from build123d import *

# Parameters (mm, degrees)
SKETCH1_W             = 152.4
SKETCH1_H             = 38.1
BOSS_EXTRUDE1_DEPTH   = 6.35
CAVITY1_START         = -18.462835622
CAVITY1_OUTLINE_W     = 6.35
CAVITY1_OUTLINE_H     = 6.35
CAVITY1_OUTLINE_W_2   = 6.2484
CAVITY1_DEPTH         = 12.7
CAVITY1_START_2       = 6.937164378
CAVITY1_2_OUTLINE_W   = 6.35
CAVITY1_2_OUTLINE_H   = 6.35
CAVITY1_2_OUTLINE_W_2 = 6.2484
CAVITY1_2_DEPTH       = 12.7
CAVITY1_START_3       = 32.337164378
CAVITY1_3_OUTLINE_W   = 6.35
CAVITY1_3_OUTLINE_H   = 6.35
CAVITY1_3_OUTLINE_W_2 = 6.2484
CAVITY1_3_DEPTH       = 12.7
CAVITY1_START_4       = 57.737164378
CAVITY1_4_OUTLINE_W   = 6.35
CAVITY1_4_OUTLINE_H   = 6.35
CAVITY1_4_OUTLINE_W_2 = 6.2484
CAVITY1_4_DEPTH       = 12.7
CAVITY1_START_5       = 83.137164378
CAVITY1_5_OUTLINE_W   = 6.35
CAVITY1_5_OUTLINE_H   = 6.35
CAVITY1_5_OUTLINE_W_2 = 6.2484
CAVITY1_5_DEPTH       = 12.7
CAVITY1_START_6       = -37.512835622
CAVITY1_6_OUTLINE_W   = 9.525
CAVITY1_6_OUTLINE_H   = 6.35
CAVITY1_6_DEPTH       = 6.35
CAVITY1_START_7       = 108.537164378
CAVITY1_7_OUTLINE_W   = 9.525
CAVITY1_7_OUTLINE_H   = 6.35
CAVITY1_7_DEPTH       = 6.35
SKETCH2_R             = 7.9375
CUT_EXTRUDE1_DEPTH    = 166.74710148
LPATTERN1_COUNT       = 5
LPATTERN1_PITCH       = 25.4


# Read off the part's stored shape, not the designer's step: Cavity1
with BuildPart() as part:
    # Sketch1 → Boss-Extrude1 (new body)
    with BuildSketch(Plane.XY):
        with Locations((38.687164378, -100.250958128)):
            Rectangle(SKETCH1_W, SKETCH1_H)
    extrude(amount=BOSS_EXTRUDE1_DEPTH)

    # Cavity1 outline → Cavity1 (cut)
    with BuildSketch(Plane.YZ.offset(CAVITY1_START)):
        with Locations((-84.375958128, 3.175)):
            Rectangle(CAVITY1_OUTLINE_W, CAVITY1_OUTLINE_H)
        with Locations((-116.176758128, 3.175)):
            Rectangle(CAVITY1_OUTLINE_W_2, CAVITY1_OUTLINE_H)
    extrude(amount=CAVITY1_DEPTH, mode=Mode.SUBTRACT)

    # Cavity1 2 outline → Cavity1 2 (cut)
    with BuildSketch(Plane.YZ.offset(CAVITY1_START_2)):
        with Locations((-84.375958128, 3.175)):
            Rectangle(CAVITY1_2_OUTLINE_W, CAVITY1_2_OUTLINE_H)
        with Locations((-116.176758128, 3.175)):
            Rectangle(CAVITY1_2_OUTLINE_W_2, CAVITY1_2_OUTLINE_H)
    extrude(amount=CAVITY1_2_DEPTH, mode=Mode.SUBTRACT)

    # Cavity1 3 outline → Cavity1 3 (cut)
    with BuildSketch(Plane.YZ.offset(CAVITY1_START_3)):
        with Locations((-84.375958128, 3.175)):
            Rectangle(CAVITY1_3_OUTLINE_W, CAVITY1_3_OUTLINE_H)
        with Locations((-116.176758128, 3.175)):
            Rectangle(CAVITY1_3_OUTLINE_W_2, CAVITY1_3_OUTLINE_H)
    extrude(amount=CAVITY1_3_DEPTH, mode=Mode.SUBTRACT)

    # Cavity1 4 outline → Cavity1 4 (cut)
    with BuildSketch(Plane.YZ.offset(CAVITY1_START_4)):
        with Locations((-84.375958128, 3.175)):
            Rectangle(CAVITY1_4_OUTLINE_W, CAVITY1_4_OUTLINE_H)
        with Locations((-116.176758128, 3.175)):
            Rectangle(CAVITY1_4_OUTLINE_W_2, CAVITY1_4_OUTLINE_H)
    extrude(amount=CAVITY1_4_DEPTH, mode=Mode.SUBTRACT)

    # Cavity1 5 outline → Cavity1 5 (cut)
    with BuildSketch(Plane.YZ.offset(CAVITY1_START_5)):
        with Locations((-84.375958128, 3.175)):
            Rectangle(CAVITY1_5_OUTLINE_W, CAVITY1_5_OUTLINE_H)
        with Locations((-116.176758128, 3.175)):
            Rectangle(CAVITY1_5_OUTLINE_W_2, CAVITY1_5_OUTLINE_H)
    extrude(amount=CAVITY1_5_DEPTH, mode=Mode.SUBTRACT)

    # Cavity1 6 outline → Cavity1 6 (cut)
    with BuildSketch(Plane.YZ.offset(CAVITY1_START_6)):
        with Locations((-95.488458128, 3.175)):
            Rectangle(CAVITY1_6_OUTLINE_W, CAVITY1_6_OUTLINE_H)
        with Locations((-114.538458128, 3.175)):
            Rectangle(CAVITY1_6_OUTLINE_W, CAVITY1_6_OUTLINE_H)
    extrude(amount=CAVITY1_6_DEPTH, mode=Mode.SUBTRACT)

    # Cavity1 7 outline → Cavity1 7 (cut)
    with BuildSketch(Plane.YZ.offset(CAVITY1_START_7)):
        with Locations((-95.488458128, 3.175)):
            Rectangle(CAVITY1_7_OUTLINE_W, CAVITY1_7_OUTLINE_H)
        with Locations((-114.538458128, 3.175)):
            Rectangle(CAVITY1_7_OUTLINE_W, CAVITY1_7_OUTLINE_H)
    extrude(amount=CAVITY1_7_DEPTH, mode=Mode.SUBTRACT)

    # Sketch2 → Cut-Extrude1 (cut, through all)
    with BuildSketch(Plane.XY.offset(6.35)):
        with Locations((-12.112835622, -100.301758128)):
            Circle(SKETCH2_R)
    cut_extrude1 = extrude(amount=-CUT_EXTRUDE1_DEPTH, mode=Mode.SUBTRACT)

    # LPattern1: Cut-Extrude1 ×5
    with Locations(*[(i * LPATTERN1_PITCH, 0, 0) for i in range(1, LPATTERN1_COUNT)]):
        add(cut_extrude1, mode=Mode.SUBTRACT)


solid = part.part
The listing builds one solid part. Answer for the finished solid, in the listing's coordinates (mm). A direction names the side the tool comes from. Coordinates: 2 decimals unless noted, no trailing zeros. Order: outer loops, then holes, each group sorted by start corner. A loop starts at its lowest first (then second) coordinate and runs counter-clockwise, first axis right, second up.
Q1. For a pull along Y with two mould halves and no side action, classify faces 5 (the face through (-34, -90.726, 3)), 6 (the face through (51, -119.301, 3)), 7 (the face through (57.737, -116, 3)) as pulls with the +Y half, pulls with the -Y half, needs draft (parallel to the pull), parting line crosses it, or undercut.
Q2. A cutting plane is placed at B-B, the plane y = -97. Write down the section's boundary in (x, z).
Q3. Consider line 1 (X direction, y = -85.5, z = 0.5); line 2 (X direction, y = -95.5, z = 1.75); line 3 (Y direction, x = 38.5, z = 4). Determine where each line is inside the solid, lowest interval first.
Q4. Which of the six approach directions +Z, -Z, +X, -X, +Y, -Y give full straight-line access (tool end or side, diameter ignored) to faces 1 (the face through (57.788, -105.132, 3.219)), 2 (the face through (70.437, -84, 3)), 3 (the face through (112, -100.251, 3)), 4 (the face through (83.137, -116, 3))?
Q5. Given P1, Ø1.5, axis at x = -8, z = 3, coming from the +Y side; P2, Ø1.9, axis at y = -116.5, z = 4, coming from the -X side, each flat-ended and moving along its own axis, determine where each tip first touches the part or whether it passes through.
Q6. A cutting plane is placed at A-A, the plane y = -86. Write down the section's boundary in (x, z).
Q7. A cutting plane is placed at C-C, the plane z = 2.25. State how many separate pieces and enclosed holes the cut face has, and give its area (3 significant figures).
Answers follow:
1. face 5: undercut
1. face 6: pulls with the -Y half
1. face 7: needs draft
2. outline: (-31.16, 0) - (-19.33, 0) - (-19.33, 6.35) - (-31.16, 6.35) - close; (-4.89, 0) - (6.07, 0) - (6.07, 6.35) - (-4.89, 6.35) - close; (20.51, 0) - (31.47, 0) - (31.47, 6.35) - (20.51, 6.35) - close; (45.91, 0) - (56.87, 0) - (56.87, 6.35) - (45.91, 6.35) - close; (71.31, 0) - (82.27, 0) - (82.27, 6.35) - (71.31, 6.35) - close; (96.71, 0) - (108.54, 0) - (108.54, 6.35) - (96.71, 6.35) - close
3. line 1: x = -37.51 to -18.46, -5.76 to 6.94, 19.64 to 32.34, 45.04 to 57.74, 70.44 to 83.14, 95.84 to 114.89
3. line 2: x = -31.16 to -18.43, -5.79 to 6.97, 19.61 to 32.37, 45.01 to 57.77, 70.41 to 83.17, 95.81 to 108.54
3. line 3: y = -113.05 to -108.24, -92.37 to -87.55
4. face 1: +Z, -Z
4. face 2: +Z, -Z, +Y
4. face 3: +Z, -Z, +X
4. face 4: +Z, -Z, -Y
5. P1: stops at y = -87.55
5. P2: stops at x = -31.16
6. outline: (-37.51, 0) - (-18.46, 0) - (-18.46, 6.35) - (-37.51, 6.35) - close; (-5.76, 0) - (6.94, 0) - (6.94, 6.35) - (-5.76, 6.35) - close; (19.64, 0) - (32.34, 0) - (32.34, 6.35) - (19.64, 6.35) - close; (45.04, 0) - (57.74, 0) - (57.74, 6.35) - (45.04, 6.35) - close; (70.44, 0) - (83.14, 0) - (83.14, 6.35) - (70.44, 6.35) - close; (95.84, 0) - (114.89, 0) - (114.89, 6.35) - (95.84, 6.35) - close
7. separate pieces: 1
7. enclosed holes: 5
7. area: 3,770 mm2
